The listing builds one solid part. Answer for the finished solid, in the listing's coordinates (mm). Face numbers are marked on the shaded views. A direction names the side the tool comes from. Give positions to 0.01 mm unless a question says otherwise; leave off trailing zeros. Order: outer loops, then holes, each group sorted by start corner. A loop starts at its lowest first (then second) coordinate and runs counter-clockwise, first axis right, second up. Notation, with made-up numbers: (-11.5, 56.5) - (37.5, 56.5) arc R12 ccw to (37.5, 63.5) - close; hole circle Ø9 at (55.5, -6). An arc over 180 degrees is marked (long way). Answer as a JSON object with one key per item and string values. Group by question number.
Q1. A cutting plane is placed at C-C, the plane y = 8. Give the vertices of the cut face in (x, z).
Q2. A cutting plane is placed at B-B, the plane z = 19.05. Give the vertices of the cut face in (x, y).
Q3. A cutting plane is placed at A-A, the plane x = 76.2. Give the vertices of the cut face in (y, z).
Q4. Given pin 1 (3 mm diameter, centred on x = -90.5, z = 42, fed in from -Y); pin 2 (11.5 mm diameter, centred on x = 76.2, z = 19.05, fed in from +Y), each flat-ended and moving along its own axis, determine where each tip first touches the part or whether it passes through.
Q5. A cutting plane is placed at D-D, the plane x = 18. Give the vertices of the cut face in (y, z), and give its area (3 significant figures).
Q6. The mould has two halves that part along X. Classify the marked faces 3, 4 and 5: released by +X, released by -X, zero draft, split by the parting line, or undercut.
Q7. For the marked faces 1 and 2, determine the directions among +Z, -Z, +X, -X, +Y, -Y from which every point of the face is accessible in a straight line to the end or side of a thin tool.
Q8. Consider line 1 (X direction, y = 46.75, z = 19.05); line 2 (Z direction, x = -76, y = 48); line 3 (X direction, y = 17, z = -16). Determine where each line is inside the solid, lowest interval first.
from build123d import *

# Parameters (mm, degrees)
SKETCH1_W           = 304.8
SKETCH1_H           = 127
BOSS_EXTRUDE1_DEPTH = 50.8
SKETCH2_W           = 279.4
SKETCH2_H           = 101.6
CUT_EXTRUDE1_DEPTH  = 44.45
SKETCH3_R           = 5.08
SKETCH3_R_2         = 6.35
CUT_EXTRUDE2_DEPTH  = 12.7


with BuildPart() as part:
    # Sketch1 → Boss-Extrude1 (new body)
    with BuildSketch(Plane(origin=(0, 0, 0), x_dir=(1, 0, 0), z_dir=(0, 1, 0))):
        Rectangle(SKETCH1_W, SKETCH1_H)
    extrude(amount=BOSS_EXTRUDE1_DEPTH)

    # Sketch2 → Cut-Extrude1 (cut)
    with BuildSketch(Plane.XZ):
        Rectangle(SKETCH2_W, SKETCH2_H)
    extrude(amount=-CUT_EXTRUDE1_DEPTH, mode=Mode.SUBTRACT)

    # Sketch3 → Cut-Extrude2 (cut)
    with BuildSketch(Plane(origin=(0, 50.8, 0), x_dir=(1, 0, 0), z_dir=(0, 1, 0))):
        with Locations(Location((-76.2, 19.05, 0), (0, 0, 270))):
            Circle(SKETCH3_R)
        with Locations(Location((76.2, 19.05, 0), (0, 0, 90))):
            Circle(SKETCH3_R)
        with Locations(Location((-76.2, -19.05, 0), (0, 0, 270))):
            Circle(SKETCH3_R_2)
        with Locations(Location((76.2, -19.05, 0), (0, 0, 270))):
            Circle(SKETCH3_R_2)
    extrude(amount=-CUT_EXTRUDE2_DEPTH, mode=Mode.SUBTRACT)


solid = part.part
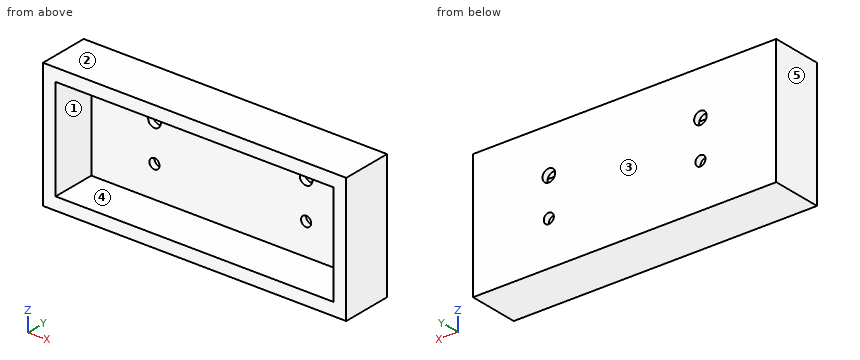
Reply:
{
 "1": {"outline": "(-152.4, -63.5) - (152.4, -63.5) - (152.4, 63.5) - (-152.4, 63.5) - close; hole (-139.7, -50.8) - (139.7, -50.8) - (139.7, 50.8) - (-139.7, 50.8) - close"},
 "2": {"outline": "(-152.4, 0) - (-139.7, 0) - (-139.7, 44.45) - (-82.55, 44.45) - (-82.55, 50.8) - (-152.4, 50.8) - close; (-69.85, 44.45) - (69.85, 44.45) - (69.85, 50.8) - (-69.85, 50.8) - close; (82.55, 44.45) - (139.7, 44.45) - (139.7, 0) - (152.4, 0) - (152.4, 50.8) - (82.55, 50.8) - close"},
 "3": {"outline": "(0, -63.5) - (50.8, -63.5) - (50.8, -24.13) - (44.45, -24.13) - (44.45, -50.8) - (0, -50.8) - close; (0, 50.8) - (44.45, 50.8) - (44.45, 25.4) - (50.8, 25.4) - (50.8, 63.5) - (0, 63.5) - close; (44.45, -13.97) - (50.8, -13.97) - (50.8, 12.7) - (44.45, 12.7) - close"},
 "4": {"pin 1": "stops at y = 44.45", "pin 2": "passes through"},
 "5": {"outline": "(0, -63.5) - (50.8, -63.5) - (50.8, 63.5) - (0, 63.5) - (0, 50.8) - (44.45, 50.8) - (44.45, -50.8) - (0, -50.8) - close", "area": "1,940 mm^2"},
 "6": {"face 3": "zero draft", "face 4": "undercut", "face 5": "released by -X"},
 "7": {"face 1": "-Y", "face 2": "+Z, +X, -X, +Y, -Y"},
 "8": {"line 1": "x = -152.4 to -82.55, -69.85 to 69.85, 82.55 to 152.4", "line 2": "z = -63.5 to -24.13, -13.97 to 12.7, 25.4 to 63.5", "line 3": "x = -152.4 to -139.7, 139.7 to 152.4"}
}
